Read the model definition and answer for the solid it produces. Units are mm, in the model's axes. A direction names the side the tool comes from. Coordinates: 2 decimals unless noted, no trailing zeros. Write each loop counter-clockwise with the first axis right and the second up, starting at its lowest first coordinate (ties: lowest second). Pieces come first, ordered by that corner, then holes. Notation, with made-up numbers: (64, -4) -> (99, -4) arc R16 ccw to (99, 6) -> close; hole circle Ø4 at (51, -8.75). An arc over 180 degrees is marked (long way). Return JSON: item names as keys, results as strings.
Autodesk Inventor part; units mm, degrees
ref_plane "YZ Plane" through (0, 0, 0) normal (1, 0, 0) x (0, 1, 0)
ref_plane "XZ Plane" through (0, 0, 0) normal (0, 1, 0) x (-1, 0, 0)
ref_plane "XY Plane" through (0, 0, 0) normal (0, 0, 1) x (1, 0, 0)
sketch "Sketch1" plane through (0, 0, 0) normal (0, 1, 0) x (-1, 0, 0)
  line L0 (12.7017, 0) -> (6.3509, -11)
  line L1 (6.3509, -11) -> (-6.3509, -11)
  line L2 (-6.3509, -11) -> (-12.7017, 0)
  line L3 (-12.7017, 0) -> (-6.3509, 11)
  line L4 (-6.3509, 11) -> (6.3509, 11)
  line L5 (6.3509, 11) -> (12.7017, 0)
  circle A0 centre (0, 0) radius 11
  circle A1 centre (0, 0) radius 4.1
  dimension "d0" = 22
  dimension "d1" = 8.2
extrude "Extrusion1" add sketch "Sketch1" along normal blind 8
sketch "Sketch2" plane through (0, 8, 0) normal (0, 1, 0) x (1, 0, 0)
  line L0 (-2.8, -8.35) -> (2.8, -8.35)
  line L1 (2.8, -8.35) -> (2.8, -5.65)
  line L2 (2.8, -5.65) -> (-2.8, -5.65)
  line L3 (-2.8, -5.65) -> (-2.8, -8.35)
  line L4 (-2.8, -8.35) -> (2.8, -5.65) construction
  line L5 (2.8, -8.35) -> (-2.8, -5.65) construction
  point P0 (0, 0)
  point P1 (0, -7)
  point P2 (0, -7)
  dimension "d4" = 2.7
  dimension "d5" = 5.6
  dimension "d8" = 7
extrude "Extrusion2" cut sketch "Sketch2" against normal blind 6.5
mirror "Mirror1" about plane through (0, 0, 0) normal (0, 0, 1) of "Extrusion2"
sketch "Sketch3" plane through (6.3509, 0, -11) normal (0, 0, -1) x (-1, 0, 0)
  circle A0 centre (6.3509, 5) radius 1.6
  line L0 (0, 0) -> (12.7017, 0)
  point P0 (6.3509, 0)
  point P1 (6.3509, 0)
  dimension "d9" = 3.2
  dimension "d10" = 5
extrude "Extrusion3" cut sketch "Sketch3" against normal through all
sketch "Sketch5" plane through (0, 0, 0) normal (0, -1, 0) x (1, 0, 0)
  circle A0 centre (0, 0) radius 11
  line L0 (6.3509, -11) -> (-6.3509, -11)
  circle A1 centre (0, 0) radius 14.2349
extrude "Extrusion5" cut sketch "Sketch5" against normal through all
sketch "Sketch6" plane through (0, 0, 0) normal (0, -1, 0) x (1, 0, 0)
  circle A0 centre (0, 0) radius 11
  circle A1 centre (0, 0) radius 4.1
extrude "Extrusion6" add sketch "Sketch6" along normal blind 2
sketch "Sketch7" plane through (0, -2, 0) normal (0, -1, 0) x (1, 0, 0)
  line L0 (-7.9674, 0) -> (-3.9837, 6.9)
  line L1 (-3.9837, 6.9) -> (3.9837, 6.9)
  line L2 (3.9837, 6.9) -> (7.9674, 0)
  line L3 (7.9674, 0) -> (3.9837, -6.9)
  line L4 (3.9837, -6.9) -> (-3.9837, -6.9)
  line L5 (-3.9837, -6.9) -> (-7.9674, 0)
  circle A0 centre (0, 0) radius 6.9
  circle A1 centre (0, 0) radius 4.1
  dimension "d19" = 13.8
extrude "Extrusion7" add sketch "Sketch7" along normal blind 10
sketch "Sketch8" plane through (0, -12, 0) normal (0, -1, 0) x (1, 0, 0)
  circle A0 centre (0, 0) radius 4.1
extrude "Extrusion8" add sketch "Sketch8" against normal blind 2
fillet "Fillet1" radius 1 6 edges at (0, -12, -6.9) (-5.9756, -12, -3.45) (-5.9756, -12, 3.45) (0, -12, 6.9) (5.9756, -12, 3.45) (5.9756, -12, -3.45)
fillet "Fillet2" radius 1 1 edges at (-11, -2, 0)
sketch "Sketch4" plane through (0, 0, 0) normal (0, -1, 0) x (1, 0, 0)
  line L0 (-2.8, -5.25) -> (2.8, -5.25)
  line L1 (2.8, -5.25) -> (2.8, -7.95)
  line L2 (2.8, -7.95) -> (-2.8, -7.95)
  line L3 (-2.8, -7.95) -> (-2.8, -5.25)
  line L4 (2.8, 5.25) -> (-2.8, 5.25)
  line L5 (-2.8, 5.25) -> (-2.8, 7.95)
  line L6 (-2.8, 7.95) -> (2.8, 7.95)
  line L7 (2.8, 7.95) -> (2.8, 5.25)
  line L8 (5.4848, -9.5) -> (-5.4848, -9.5)
  line L9 (10.9697, 0) -> (5.4848, -9.5)
  line L10 (5.4848, 9.5) -> (10.9697, 0)
  line L11 (-5.4848, 9.5) -> (5.4848, 9.5)
  line L12 (-10.9697, 0) -> (-5.4848, 9.5)
  line L13 (-5.4848, -9.5) -> (-10.9697, 0)
  circle A0 centre (0, 0) radius 4.1
properties part number "EndNut"
1. The part is cut by section D-D (y = 5). Determine the outline of the cut face in (x, z).
Taken from the geometry:
{"outline": "(-2.8, -8.35) -> (-2.8, -5.65) -> (-1.6, -5.65) -> (-1.6, -3.77) arc R4.1 cw to (-1.6, 3.77) -> (-1.6, 5.65) -> (-2.8, 5.65) -> (-2.8, 8.35) -> (-1.6, 8.35) -> (-1.6, 10.88) arc R11 ccw to (-1.6, -10.88) -> (-1.6, -8.35) -> close; (1.6, -10.88) arc R11 ccw to (1.6, 10.88) -> (1.6, 8.35) -> (2.8, 8.35) -> (2.8, 5.65) -> (1.6, 5.65) -> (1.6, 3.77) arc R4.1 cw to (1.6, -3.77) -> (1.6, -5.65) -> (2.8, -5.65) -> (2.8, -8.35) -> (1.6, -8.35) -> close"}
2. The part is cut by section C-C (x = 0). Count the separate pieces of the cut face and the enclosed holes in it, then the cut area to 3 significant figures.
Taken from the geometry:
{"separate pieces": "5", "enclosed holes": "0", "area": "148 mm2"}
3. A tool of negligible diameter and unlimited length cuts with its end or side. For faces 1 (the face through (-6.003, -6.437, 3.402)), 2 (the face through (-5.948, -6.437, -3.498)), 3 (the face through (6.003, -6.437, -3.402)), 4 (the face through (0, 3, -5.65)), from which of +Z, -Z, +X, -X, +Y, -Y can it reach the whole face along a straight path? Write none if from no direction.
Taken from the geometry:
{"face 1": "+Z, -X, -Y", "face 2": "-Z, -X, -Y", "face 3": "-Z, +X, -Y", "face 4": "+Y"}
4. Consider L1, parallel to Y at x = 0, z = 4.45; L2, parallel to X at y = 2.5, z = 0; L3, parallel to Z at x = 0, y = -8. Determine where each line is inside the solid, lowest interval first.
Taken from the geometry:
{"L1": "y = -12 to 3.4, 6.6 to 8", "L2": "x = -11 to -4.1, 4.1 to 11", "L3": "z = -6.9 to -4.1, 4.1 to 6.9"}
5. The part is cut by section B-B (y = 2.5). Determine the outline of the cut face in (x, z).
Taken from the geometry:
{"outline": "circle Ø22 at (0, 0); hole circle Ø8.2 at (0, 0); hole (-2.8, -8.35) -> (2.8, -8.35) -> (2.8, -5.65) -> (-2.8, -5.65) -> close; hole (-2.8, 5.65) -> (2.8, 5.65) -> (2.8, 8.35) -> (-2.8, 8.35) -> close"}
6. For a pull along X with two mould halves and no side action, classify faces 5 (the face through (0, -12, 0)), 6 (the face through (-5.756, -11.699, -3.259)), 7 (the face through (2.8, 5, -7)), 8 (the face through (5.948, -6.437, 3.498)) as +X half, -X half, draft (parallel to the pull), parting line (faces both ways), or undercut.
Taken from the geometry:
{"face 5": "draft", "face 6": "-X half", "face 7": "undercut", "face 8": "+X half"}
7. Flat-ended cylindrical pins translate along their axes: pin 1 Ø5 at (x, y) = (0, 5) entering from -Z; pin 2 Ø1.3 at (y, z) = (4.5, 6.5) entering from -X; pin 3 Ø4 at (x, y) = (0.5, -7) entering from +Z; pin 4 Ø2 at (y, z) = (6, -7) entering from +X. Find the tip coordinate at first contact, or state that the pin passes through.
Taken from the geometry:
{"pin 1": "stops at z = -11", "pin 2": "stops at x = -9.32", "pin 3": "stops at z = 6.9", "pin 4": "stops at x = 9.22"}
8. The part is cut by section A-A (y = -9.5). Determine the outline of the cut face in (x, z).
Taken from the geometry:
{"outline": "(-7.97, 0) -> (-3.98, -6.9) -> (3.98, -6.9) -> (7.97, 0) -> (3.98, 6.9) -> (-3.98, 6.9) -> close; hole circle Ø8.2 at (0, 0)"}
